Verification items for the finished model (mm, model axes). A direction names the side the tool comes from. Round coordinates to 2 decimals unless told otherwise and drop trailing zeros. Write each loop counter-clockwise with the first axis right and the second up, starting at its lowest first coordinate (ties: lowest second). Pieces come first, ordered by that corner, then holes. Notation, with made-up numbers: (77.5, 58.5) -> (101.5, 58.5) arc R22 cw to (101.5, 77.5) -> close; hole circle Ø2 at (43.5, 32.5). An arc over 180 degrees is marked (long way). Answer as a JSON object with one key per item and string values. Group by question number.
(1) Sectioned sample at B-B on z = -25.5. Count the separate pieces of the cut face and the enclosed holes in it, and give its area (3 significant figures).
(2) Gauge pin test, flat ends, axial feed: pin 1 Ø1.3 at (y, z) = (-14, -38) entering from +X; pin 2 Ø2 at (y, z) = (2.5, -81.5) entering from +X; pin 3 Ø0.6 at (y, z) = (14.5, -35) entering from -X; pin 4 Ø1.5 at (x, y) = (11.5, -3.5) entering from -Z. Record the tip position at first contact, or that the pin passes through.
(3) Set-up check for faces 1 (the face through (-1, -5, -100)), 2 (the face through (-12.793, -7, -49)): record each of +Z, -Z, +X, -X, +Y, -Y from which the full face is reachable in a straight line by a thin tool's end or side.
(4) Draft check along X on faces 3 (the face through (-1, -5, 0)), 4 (the face through (-5.95, 0, -49)), 5 (the face through (14.48, -14.45, -49.3)), 6 (the face through (-12, -9.66, -49)). Enter one of: released by +X, released by -X, zero draft, split by the parting line, or undercut.
(5) Scan lines: L1, parallel to Y at x = 12, z = -24; L2, parallel to X at y = 7.25, z = -48.5; L3, parallel to Y at x = -4.25, z = -16.5. Record each from-to range of solid material in increasing order. Write a range as from..to.
(6) Sectioned sample at A-A on y = -7.25. Record the cut outline in (x, z), and give its area (3 significant figures).
```python
from build123d import *

# Parameters (mm, degrees)
SKETCH1_W           = 11.9
SKETCH1_H           = 5.95
BOSS_EXTRUDE1_DEPTH = 100
CUT_EXTRUDE1_DEPTH  = 101


with BuildPart() as part:
    # Sketch1 → Boss-Extrude1 (new body)
    with BuildSketch(Plane.XY):
        with BuildLine():
            Line((-4.350229073, 14.992640687), (-13.192640687, 14.992640687))
            ThreePointArc((-13.192640687, 14.992640687), (-14.465432893, 14.465432893), (-14.992640687, 13.192640687))
            Line((-14.992640687, 13.192640687), (-14.992640687, 4.350229073))
            Line((-14.992640687, 4.350229073), (-13.792640687, 4.350229073))
            ThreePointArc((-13.792640687, 4.350229073), (-13.085533906, 4.643122292), (-12.792640687, 5.350229073))
            Line((-12.792640687, 5.350229073), (-12.792640687, 8.460229073))
            Line((-12.792640687, 8.460229073), (-8.460229073, 8.460229073))
            Line((-8.460229073, 8.460229073), (-8.460229073, 12.792640687))
            Line((-8.460229073, 12.792640687), (-5.350229073, 12.792640687))
            ThreePointArc((-5.350229073, 12.792640687), (-4.643122292, 13.085533906), (-4.350229073, 13.792640687))
            Line((-4.350229073, 13.792640687), (-4.350229073, 14.992640687))
        make_face()
        with BuildLine():
            Line((-10.660229073, 13.792640687), (-12.792640687, 13.792640687))
            ThreePointArc((-12.792640687, 13.792640687), (-13.499747468, 13.499747468), (-13.792640687, 12.792640687))
            Line((-13.792640687, 12.792640687), (-13.792640687, 10.660229073))
            ThreePointArc((-13.792640687, 10.660229073), (-13.499747468, 9.953122292), (-12.792640687, 9.660229073))
            Line((-12.792640687, 9.660229073), (-10.660229073, 9.660229073))
            ThreePointArc((-10.660229073, 9.660229073), (-9.953122292, 9.953122292), (-9.660229073, 10.660229073))
            Line((-9.660229073, 10.660229073), (-9.660229073, 12.792640687))
            ThreePointArc((-9.660229073, 12.792640687), (-9.953122292, 13.499747468), (-10.660229073, 13.792640687))
        make_face(mode=Mode.SUBTRACT)
        Polygon((-5.95, 4.217588386), (-5.95, 5.95), (-4.217588386, 5.95), (-8.460229073, 10.192640687), (-8.460229073, 8.460229073), (-10.192640687, 8.460229073), align=None)
        with Locations((0, 2.975)):
            Rectangle(SKETCH1_W, SKETCH1_H)
        Polygon((8.460229073, 10.192640687), (4.217588386, 5.95), (5.95, 5.95), (5.95, 4.217588386), (10.192640687, 8.460229073), (8.460229073, 8.460229073), align=None)
        with BuildLine():
            Line((12.792640687, 8.460229073), (12.792640687, 5.350229073))
            ThreePointArc((12.792640687, 5.350229073), (13.085533906, 4.643122292), (13.792640687, 4.350229073))
            Line((13.792640687, 4.350229073), (14.992640687, 4.350229073))
            Line((14.992640687, 4.350229073), (14.992640687, 13.192640687))
            ThreePointArc((14.992640687, 13.192640687), (14.465432893, 14.465432893), (13.192640687, 14.992640687))
            Line((13.192640687, 14.992640687), (4.350229073, 14.992640687))
            Line((4.350229073, 14.992640687), (4.350229073, 13.792640687))
            ThreePointArc((4.350229073, 13.792640687), (4.643122292, 13.085533906), (5.350229073, 12.792640687))
            Line((5.350229073, 12.792640687), (8.460229073, 12.792640687))
            Line((8.460229073, 12.792640687), (8.460229073, 8.460229073))
            Line((8.460229073, 8.460229073), (12.792640687, 8.460229073))
        make_face()
        with BuildLine():
            ThreePointArc((9.660229073, 10.660229073), (9.953122292, 9.953122292), (10.660229073, 9.660229073))
            Line((10.660229073, 9.660229073), (12.792640687, 9.660229073))
            ThreePointArc((12.792640687, 9.660229073), (13.499747468, 9.953122292), (13.792640687, 10.660229073))
            Line((13.792640687, 10.660229073), (13.792640687, 12.792640687))
            ThreePointArc((13.792640687, 12.792640687), (13.499747468, 13.499747468), (12.792640687, 13.792640687))
            Line((12.792640687, 13.792640687), (10.660229073, 13.792640687))
            ThreePointArc((10.660229073, 13.792640687), (9.953122292, 13.499747468), (9.660229073, 12.792640687))
            Line((9.660229073, 12.792640687), (9.660229073, 10.660229073))
        make_face(mode=Mode.SUBTRACT)
    extrude(amount=-BOSS_EXTRUDE1_DEPTH)

    # Mirror1: part across plane


with BuildPart() as part_1:
    add(part.part)
    add(part.part.mirror(Plane(origin=(0, 0, -100), x_dir=(0, 0, 1), z_dir=(0, -1, 0))))

    # Sketch2 → Cut-Extrude1 (cut, through all)
    with BuildSketch(Plane.XY):
        with BuildLine():
            Line((-4.631549417, 3.075914498), (-3.16821753, 1.612582612))
            ThreePointArc((-3.16821753, 1.612582612), (-2.513764607, 2.513764607), (-1.612582612, 3.16821753))
            Line((-1.612582612, 3.16821753), (-3.075914498, 4.631549417))
            Line((-3.075914498, 4.631549417), (-4.631549417, 3.075914498))
        make_face()
        with BuildLine():
            Line((-3.16821753, 1.612582612), (-1.555634919, 0))
            Line((-1.555634919, 0), (0, 1.555634919))
            Line((0, 1.555634919), (-1.612582612, 3.16821753))
            ThreePointArc((-1.612582612, 3.16821753), (-2.513764607, 2.513764607), (-3.16821753, 1.612582612))
        make_face()
        with BuildLine():
            ThreePointArc((-3.16821753, 1.612582612), (-3.555, 0), (-3.16821753, -1.612582612))
            Line((-3.16821753, -1.612582612), (-1.555634919, 0))
            Line((-1.555634919, 0), (-3.16821753, 1.612582612))
        make_face()
        with BuildLine():
            Line((-4.631549417, -3.075914498), (-3.075914498, -4.631549417))
            Line((-3.075914498, -4.631549417), (-1.612582612, -3.16821753))
            ThreePointArc((-1.612582612, -3.16821753), (-2.513764607, -2.513764607), (-3.16821753, -1.612582612))
            Line((-3.16821753, -1.612582612), (-4.631549417, -3.075914498))
        make_face()
        with BuildLine():
            ThreePointArc((-3.16821753, -1.612582612), (-2.513764607, -2.513764607), (-1.612582612, -3.16821753))
            Line((-1.612582612, -3.16821753), (0, -1.555634919))
            Line((0, -1.555634919), (-1.555634919, 0))
            Line((-1.555634919, 0), (-3.16821753, -1.612582612))
        make_face()
        with BuildLine():
            Line((0, -1.555634919), (-1.612582612, -3.16821753))
            ThreePointArc((-1.612582612, -3.16821753), (0, -3.555), (1.612582612, -3.16821753))
            Line((1.612582612, -3.16821753), (0, -1.555634919))
        make_face()
        with BuildLine():
            Line((1.555634919, 0), (0, -1.555634919))
            Line((0, -1.555634919), (1.612582612, -3.16821753))
            ThreePointArc((1.612582612, -3.16821753), (2.513764607, -2.513764607), (3.16821753, -1.612582612))
            Line((3.16821753, -1.612582612), (1.555634919, 0))
        make_face()
        with BuildLine():
            Line((3.16821753, 1.612582612), (1.555634919, 0))
            Line((1.555634919, 0), (3.16821753, -1.612582612))
            ThreePointArc((3.16821753, -1.612582612), (3.456952294, -0.829159719), (3.555, 0))
            ThreePointArc((3.555, 0), (3.456952294, 0.829159719), (3.16821753, 1.612582612))
        make_face()
        Polygon((-1.555634919, 0), (0, -1.555634919), (1.555634919, 0), (0, 1.555634919), align=None)
        with BuildLine():
            Line((0, 1.555634919), (1.555634919, 0))
            Line((1.555634919, 0), (3.16821753, 1.612582612))
            ThreePointArc((3.16821753, 1.612582612), (2.513764607, 2.513764607), (1.612582612, 3.16821753))
            Line((1.612582612, 3.16821753), (0, 1.555634919))
        make_face()
        with BuildLine():
            Line((-1.612582612, 3.16821753), (0, 1.555634919))
            Line((0, 1.555634919), (1.612582612, 3.16821753))
            ThreePointArc((1.612582612, 3.16821753), (0, 3.555), (-1.612582612, 3.16821753))
        make_face()
        with BuildLine():
            ThreePointArc((1.612582612, 3.16821753), (2.513764607, 2.513764607), (3.16821753, 1.612582612))
            Line((3.16821753, 1.612582612), (4.631549417, 3.075914498))
            Line((4.631549417, 3.075914498), (3.075914498, 4.631549417))
            Line((3.075914498, 4.631549417), (1.612582612, 3.16821753))
        make_face()
        with BuildLine():
            ThreePointArc((3.16821753, -1.612582612), (2.513764607, -2.513764607), (1.612582612, -3.16821753))
            Line((1.612582612, -3.16821753), (3.075914498, -4.631549417))
            Line((3.075914498, -4.631549417), (4.631549417, -3.075914498))
            Line((4.631549417, -3.075914498), (3.16821753, -1.612582612))
        make_face()
    extrude(amount=-CUT_EXTRUDE1_DEPTH, mode=Mode.SUBTRACT)


solid = part_1.part
```
Computed values:
{
 "1": {"separate pieces": "1", "enclosed holes": "5", "area": "305 mm2"},
 "2": {"pin 1": "x = 14.99", "pin 2": "x = 5.95", "pin 3": "x = -14.68", "pin 4": "through"},
 "3": {"face 1": "-Z, +X, -X, +Y, -Y", "face 2": "+Z, -Z"},
 "4": {"face 3": "zero draft", "face 4": "released by -X", "face 5": "released by +X", "face 6": "undercut"},
 "5": {"L1": "-14.99..-13.79, -9.66..-8.46, 8.46..9.66, 13.79..14.99", "L2": "-14.99..-12.79, -8.98..-5.52, 5.52..8.98, 12.79..14.99", "L3": "-5.98..-3.46, -2.69..2.69, 3.46..5.98"},
 "6": {"outline": "(-14.99, -100) -> (-12.79, -100) -> (-12.79, 0) -> (-14.99, 0) -> close; (-8.98, -100) -> (-5.52, -100) -> (-5.52, 0) -> (-8.98, 0) -> close; (5.52, -100) -> (8.98, -100) -> (8.98, 0) -> (5.52, 0) -> close; (12.79, -100) -> (14.99, -100) -> (14.99, 0) -> (12.79, 0) -> close", "area": "1,130 mm2"}
}
